The model under review builds one solid part; all positions refer to its coordinate system, in mm. Face numbers are marked on the shaded views. A direction names the side the tool comes from. Round coordinates to 2 decimals unless told otherwise and drop trailing zeros. Loops run counter-clockwise (first coordinate to the right, second up) from the corner with the lowest first, then second, coordinate; pieces in that order, holes last. Notation, with made-up numbers: M 80.5,64.25 L 89.5,64.25 A26 ccw 89.5,95.25 Z; hole C 29.5,19.25 d1. An arc over 180 degrees is marked long. Use a Markdown table: item, result. Add a question column.
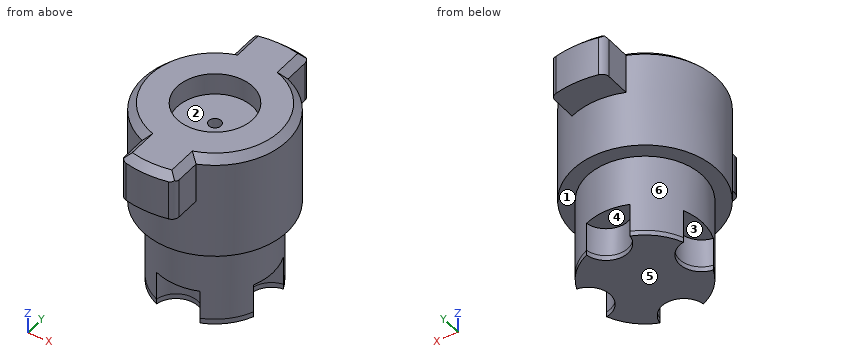
Autodesk Inventor part; units mm, degrees
ref_plane "YZ Plane" through (0, 0, 0) normal (1, 0, 0) x (0, 1, 0)
ref_plane "XZ Plane" through (0, 0, 0) normal (0, 1, 0) x (-1, 0, 0)
ref_plane "XY Plane" through (0, 0, 0) normal (0, 0, 1) x (1, 0, 0)
sketch "スケッチ1" plane through (0, 0, 0) normal (0, 0, 1) x (1, 0, 0)
  circle A0 centre (0, 0) radius 10
  dimension "d0" = 20
extrude "押し出し1" add sketch "スケッチ1" along normal blind 6.5
sketch "スケッチ2" plane through (0, 0, 0) normal (0, 0, -1) x (-1, 0, 0)
  arc A0 (3.75, 13.4884) -> (-3.75, 13.4884) centre (0, 0) ccw
  arc A1 (-3.75, -13.4884) -> (3.75, -13.4884) centre (0, 0) ccw
  circle A2 centre (0, 0) radius 10
  line L0 (-3.75, 13.4884) -> (-3.75, -13.4884)
  line L1 (3.75, -13.4884) -> (3.75, 13.4884)
  line L2 (0, -19.6) -> (0, 19.6)
  line L3 (14, 0) -> (-14, 0)
  point P0 (0, 14)
  point P1 (0, -14)
  point P2 (-3.75, 0)
  dimension "d3" = 14
  dimension "d4" = 7.5
extrude "押し出し2" add sketch "スケッチ2" against normal up to surface (6.5 mm away) contours L1 A2 L2 A0 | L2 A2 L0 A0 | L1 L3 L2 A2 | L2 L3 L0 A2 | L1 A2 L2 L3 | L2 A2 L0 L3 | L1 A1 L2 A2 | L2 A1 L0 A2
chamfer "面取り1" distance 1 angle 45 8 edges at (-10, 0, 6.5) (10, 0, 6.5) (-3.75, 11.3793, 6.5) (0, 14, 6.5) (3.75, 11.3793, 6.5) (3.75, -11.3793, 6.5) (0, -14, 6.5) (-3.75, -11.3793, 6.5)
fillet "フィレット1" radius 1 4 edges at (-3.75, -13.4884, 2.75) (3.75, -13.4884, 2.75) (3.75, 13.4884, 2.75) (-3.75, 13.4884, 2.75)
sketch "スケッチ4" plane through (0, 0, 0) normal (0, 0, -1) x (-1, 0, 0)
  circle A0 centre (0, 0) radius 8
  dimension "d14" = 16
extrude "押し出し4" add sketch "スケッチ4" along normal blind 19
sketch "スケッチ5" plane through (0, 0, 6.5) normal (0, 0, 1) x (1, 0, 0)
  circle A0 centre (0, 0) radius 5.25
  dimension "d17" = 10.5
extrude "押し出し5" cut sketch "スケッチ5" against normal blind 3
sketch "スケッチ6" plane through (0, 0, -19) normal (0, 0, -1) x (-1, 0, 0)
  circle A0 centre (0, 7.85) radius 3.05
  line L0 (14, 0) -> (-14, 0)
  line L1 (0, -19.6) -> (0, 19.6)
  point P0 (0, 0)
  dimension "d20" = 6.1
  dimension "d21" = 7.85
extrude "押し出し6" cut sketch "スケッチ6" against normal blind 4
pattern_circular "円形状パターン1" count 4 over 360 about axis through (0, 0, -10) along (0, 0, 1) of "押し出し6"
sketch "スケッチ7" plane through (0, 0, 0) normal (0, 0, -1) x (-1, 0, 0)
  circle A0 centre (0, 0) radius 5.25
  circle A1 centre (0, 0) radius 10
  point P0 (-3.75, -9.2702)
extrude "押し出し7" add sketch "スケッチ7" along normal blind 8
sketch "スケッチ8" plane through (0, 0, -19) normal (0, 0, -1) x (-1, 0, 0)
  arc A0 (-7.4089, -3.0179) -> (-7.4089, 3.0179) centre (-7.85, 0) ccw
  arc A1 (-7.4089, -3.0179) -> (-3.0179, -7.4089) centre (0, 0) ccw
  arc A2 (3.0179, -7.4089) -> (-3.0179, -7.4089) centre (0, -7.85) ccw
  arc A3 (3.0179, -7.4089) -> (7.4089, -3.0179) centre (0, 0) ccw
  arc A4 (7.4089, 3.0179) -> (7.4089, -3.0179) centre (7.85, 0) ccw
  arc A5 (7.4089, 3.0179) -> (3.0179, 7.4089) centre (0, 0) ccw
  arc A6 (-3.0179, 7.4089) -> (3.0179, 7.4089) centre (0, 7.85) ccw
  arc A7 (-3.0179, 7.4089) -> (-7.4089, 3.0179) centre (0, 0) ccw
extrude "押し出し8" add sketch "スケッチ8" along normal blind 0.708
sketch "スケッチ9" plane through (0, 0, 3.5) normal (0, 0, 1) x (1, 0, 0)
  circle A0 centre (0, 0) radius 0.85
  dimension "d31" = 1.7
extrude "押し出し9" cut sketch "スケッチ9" against normal blind 12
properties part number "conecter"
(1) Draft analysis for pull direction X (two halves, no side actions). For the marked faces 4, 5 and 6, state which applies: released by +X, released by -X, zero draft, split by the parting line, or undercut.
(2) Insertion check: pin 1 Ø3 at (x, y) = (-1, -7) entering from -Z; pin 2 Ø2 at (x, z) = (3.5, -2.5) entering from -Y; pin 3 Ø4 at (y, z) = (-5.5, -4) entering from +X. Each pin has a flat end and moves straight along its axis. Give the tip position at first contact, or say it passes through.
(3) Consider section D-D, the plane z = -6.25. Give the boundary of the cut face in (x, y).
(4) Consider section B-B, the plane z = -15.75. Give the boundary of the cut face in (x, y).
(5) To check wall thickness, follow probe 1 along Y at (x, z) = (0, 4.3); probe 2 along Y at (x, z) = (0, -6); probe 3 along Z at (x, y) = (3.5, -7.5). State the ranges of each line that lie inside material, in increasing order.
(6) Consider section A-A, the plane z = 2.5. Give the boundary of the cut face in (x, y), then the cut area to 3 significant figures.
(7) For the marked faces 1, 2 and 3, list the 3-axis set-ups (+Z, -Z, +X, -X, +Y, -Y) from which the entire face can be reached by the end or side of a thin tool; tool diameter is ignored.
(8) Consider section C-C, the plane x = 0. Give the boundary of the cut face in (y, z), then the cut area to 3 significant figures.
Found:
| question | item | result |
|---|---|---|
| 1 | face 4 | undercut |
| 1 | face 5 | zero draft |
| 1 | face 6 | split by the parting line |
| 2 | pin 1 | stops at z = -15 |
| 2 | pin 2 | stops at y = -9.68 |
| 2 | pin 3 | stops at x = 9.37 |
| 3 | outline | C 0,0 d20; hole C 0,0 d1.7 |
| 4 | outline | M -7.41,-3.02 A8 ccw -3.02,-7.41 A3.05 cw 3.02,-7.41 A8 ccw 7.41,-3.02 A3.05 cw 7.41,3.02 A8 ccw 3.02,7.41 A3.05 cw -3.02,7.41 A8 ccw -7.41,3.02 A3.05 cw Z |
| 5 | probe 1 | y = -14 to -5.25, 5.25 to 14 |
| 5 | probe 2 | y = -10 to -0.85, 0.85 to 10 |
| 5 | probe 3 | z = -8 to 6.5 |
| 6 | outline | M -3.75,-12.71 A1 ccw -2.96,-13.68 A14 ccw 2.96,-13.68 A1 ccw 3.75,-12.71 L 3.75,-9.27 A10 ccw 3.75,9.27 L 3.75,12.71 A1 ccw 2.96,13.68 A14 ccw -2.96,13.68 A1 ccw -3.75,12.71 L -3.75,9.27 A10 ccw -3.75,-9.27 Z; hole C 0,0 d1.7 |
| 6 | area | 372 mm^2 |
| 7 | face 1 | -Z |
| 7 | face 2 | +Z |
| 7 | face 3 | -Z, -X |
| 8 | outline | M -14,0 L -10,0 L -10,-8 L -8,-8 L -8,-15 L -4.8,-15 L -4.8,-19.71 L 4.8,-19.71 L 4.8,-15 L 8,-15 L 8,-8 L 10,-8 L 10,0 L 14,0 L 14,5.5 L 13,6.5 L 5.25,6.5 L 5.25,3.5 L 0.85,3.5 L 0.85,-8.5 L -0.85,-8.5 L -0.85,3.5 L -5.25,3.5 L -5.25,6.5 L -13,6.5 L -14,5.5 Z |
| 8 | area | 446 mm^2 |
